Study the drawing (mm; zero at the part's minimum x, y, z) and answer. A direction names the side the tool comes from. Round coordinates to 2 decimals unless told otherwise and drop trailing zeros. Order: outer loops, then holes, each group sorted by start corner. A loop starts at its lowest first (then second) coordinate and runs counter-clockwise, first axis right, second up. Notation, with made-up numbers: (39, -12) - (73, -12) arc R14 ccw to (73, 6) - close; hole circle Ø4 at (40.25, 34.5). An arc over 180 degrees is marked (long way). Use one line per item in the form item = value. Start each with the question number.
Q1. The part is cut by section A-A on z = 2.75. Determine the outline of the cut face in (x, y), plus the area to 3 significant figures.
Q2. The part is cut by section B-B on x = 28. Determine the outline of the cut face in (y, z), plus the area to 3 significant figures.
Q3. Find the intervals of material crossed by line 1 (X direction, y = 2.65, z = 5.75); line 2 (Y direction, x = 23, z = 3); line 3 (Z direction, x = 58.5, y = 2.7), in increasing order. Write a range as [from, to].
Q4. Given P1, Ø0.9, axis at y = 2, z = 7.5, coming from the -X side; P2, Ø1.5, axis at y = 2, z = 6.5, coming from the +X side; P3, Ø3, axis at x = 3, z = 9, coming from the -Y side, each flat-ended and moving along its own axis, determine where each tip first touches the part or whether it passes through.
Q5. Which of the six approach directions +Z, -Z, +X, -X, +Y, -Y give full straight-line access (tool end or side, diameter ignored) to the marked faces 1, 2 and 3?
Q6. The part is cut by section C-C on y = 0.7. Determine the outline of the cut face in (x, z), plus the area to 3 significant figures.
Q7. The part is cut by section D-D on z = 9.75. Determine the outline of the cut face in (x, y).
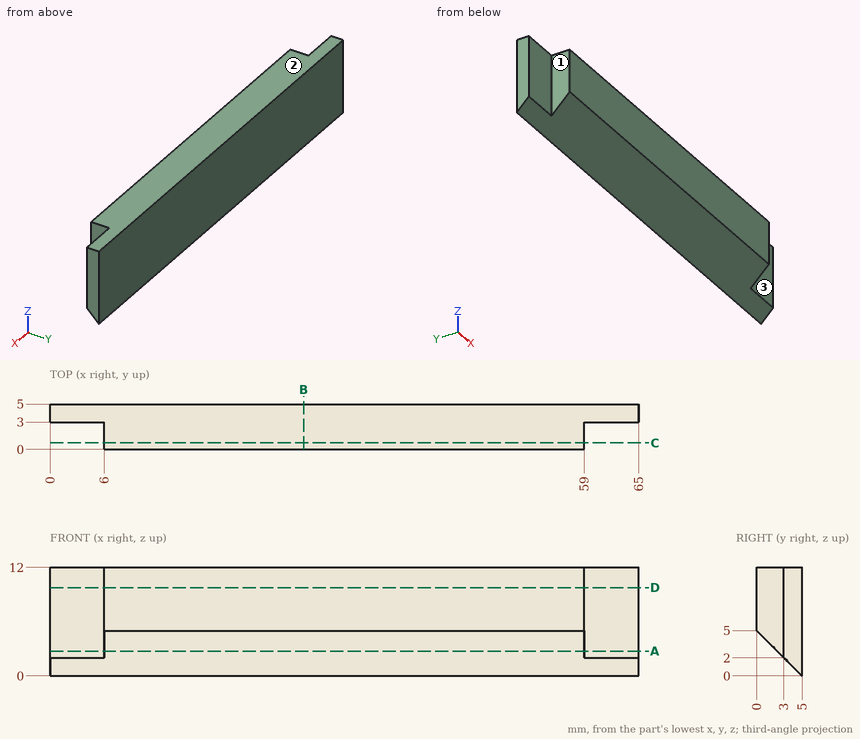
Found:
q1.outline = (0, 3) - (6, 3) - (6, 2.25) - (59, 2.25) - (59, 3) - (65, 3) - (65, 5) - (0, 5) - close
q1.area = 170 mm²
q2.outline = (0, 5) - (5, 0) - (5, 12) - (0, 12) - close
q2.area = 47.5 mm²
q3.line_1 = [6, 59]
q3.line_2 = [2, 5]
q3.line_3 = [2.3, 12]
q4.P1 = 6
q4.P2 = 59
q4.P3 = 3
q5.face_1 = +Z, -Z, -X, -Y
q5.face_2 = +Z, +X, -X, +Y, -Y
q5.face_3 = +Z, -Z, +X, -Y
q6.outline = (6, 4.3) - (59, 4.3) - (59, 12) - (6, 12) - close
q6.area = 408 mm²
q7.outline = (0, 3) - (6, 3) - (6, 0) - (59, 0) - (59, 3) - (65, 3) - (65, 5) - (0, 5) - close
